Source: CAD feature listing. Evaluate the final solid. Frame: model axes, mm. Face numbers are marked on the shaded views. A direction names the side the tool comes from. Give positions to 0.01 mm unless a question says otherwise; leave off trailing zeros. Order: outer loops, then holes, each group sorted by start corner. A loop starts at its lowest first (then second) coordinate and runs counter-clockwise, first axis right, second up.
from build123d import *

# Parameters (mm, degrees)
BOSS_EXTRUDE1_DEPTH = 20


with BuildPart() as part:
    # Sketch1 → Boss-Extrude1 (new, symmetric)
    with BuildSketch(Plane(origin=(0, 0, 0), x_dir=(1, 0, 0), z_dir=(0, 1, 0))):
        with BuildLine():
            Line((13.7, 0), (13.7, 6))
            ThreePointArc((13.7, 6), (16.043145751, 11.656854249), (21.7, 14))
            Line((21.7, 14), (30.7, 14))
            Line((30.7, 14), (30.7, 12))
            Line((30.7, 12), (21.7, 12))
            ThreePointArc((21.7, 12), (17.457359313, 10.242640687), (15.7, 6))
            Line((15.7, 6), (15.7, 0))
            ThreePointArc((15.7, 0), (0, -15.7), (-15.7, 0))
            Line((-15.7, 0), (-15.7, 6))
            ThreePointArc((-15.7, 6), (-17.457359313, 10.242640687), (-21.7, 12))
            Line((-21.7, 12), (-30.7, 12))
            Line((-30.7, 12), (-30.7, 14))
            Line((-30.7, 14), (-21.7, 14))
            ThreePointArc((-21.7, 14), (-16.043145751, 11.656854249), (-13.7, 6))
            Line((-13.7, 6), (-13.7, 0))
            ThreePointArc((-13.7, 0), (0, -13.7), (13.7, 0))
        make_face()
    extrude(amount=BOSS_EXTRUDE1_DEPTH, both=True)


solid = part.part
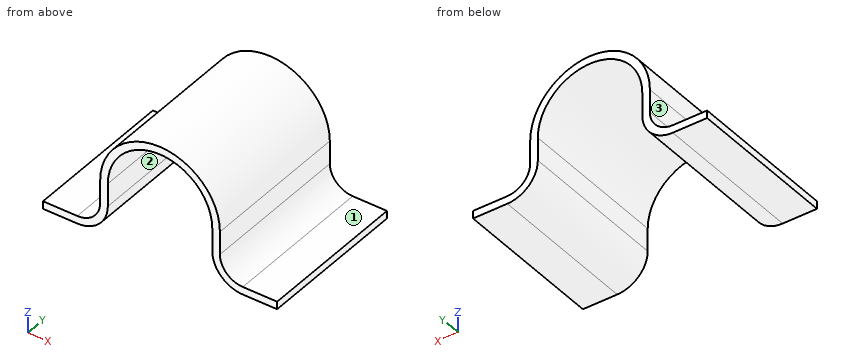
(1) Access query for the marked faces 1, 2 and 3. Directions: +Z, -Z, +X, -X, +Y, -Y. A direction counts if a zero-diameter tool reaches every point of the face in a straight line with its end or side. Return the directions, or none.
(2) Section A-A, the plane z = -2. Return loops of the section in (x, y).
(3) Pin query (flat end, axial travel): pin 1 Ø2 at (y, z) = (14, 3) entering from +X; pin 2 Ø6 at (y, z) = (-13, 12.5) entering from +X; pin 3 Ø6 at (x, y) = (-14, 11) entering from +Z. Return the tip coordinate at first contact, or that it passes through.
(4) Section D-D, the plane z = 5. Return loops of the section in (x, y) (3 decimals), plus the area to 3 significant figures.
(5) Section C-C, the plane x = 0. Return loops of the section in (y, z), plus the area to 3 significant figures.
(6) Section B-B, the plane y = 5.5. Return loops of the section in (x, z).
(7) Line query: line 1 along X through (y, z) = (-10.5, 0.5); line 2 along Z through (x, y) = (-0.5, 9); line 3 along X through (y, z) = (0.5, -10.75). Output: solid intervals per line, ascending.
Checks:
1. face 1: +Z, +X, +Y, -Y
1. face 2: -Z, +Y, -Y
1. face 3: +Z, -X, +Y, -Y
2. outline: (-15.7, -20) - (-13.7, -20) - (-13.7, 20) - (-15.7, 20) - close; (13.7, -20) - (15.7, -20) - (15.7, 20) - (13.7, 20) - close
3. pin 1: stops at x = 15.57
3. pin 2: stops at x = 12.5
3. pin 3: stops at z = 11.2
4. outline: (-14.883, -20) - (-12.755, -20) - (-12.755, 20) - (-14.883, 20) - close; (12.755, -20) - (14.883, -20) - (14.883, 20) - (12.755, 20) - close
4. area: 170 mm2
5. outline: (-20, 13.7) - (20, 13.7) - (20, 15.7) - (-20, 15.7) - close
5. area: 80.0 mm2
6. outline: (-30.7, -14) - (-21.7, -14) arc R8 ccw to (-13.7, -6) - (-13.7, 0) arc R13.7 cw to (13.7, 0) - (13.7, -6) arc R8 ccw to (21.7, -14) - (30.7, -14) - (30.7, -12) - (21.7, -12) arc R6 cw to (15.7, -6) - (15.7, 0) arc R15.7 ccw to (-15.7, 0) - (-15.7, -6) arc R6 cw to (-21.7, -12) - (-30.7, -12) - close
7. line 1: x = -15.69 to -13.69, 13.69 to 15.69
7. line 2: z = 13.69 to 15.69
7. line 3: x = -18.03 to -15.26, 15.26 to 18.03
